```python
from build123d import *

# Parameters (mm, degrees)
BOSS_EXTRUDE1_DEPTH = 3.175
SKETCH2_R           = 1.5875
CUT_EXTRUDE_R_DEPTH = 216.549531721


with BuildPart() as part:
    # Sketch1 → Boss-Extrude1 (new body)
    with BuildSketch(Plane.XY):
        Polygon((0, 0), (0, 152.4), (152.4, 152.4), align=None)
    extrude(amount=BOSS_EXTRUDE1_DEPTH)

    # Sketch2 → Cut-Extrude r (cut, through all)
    with BuildSketch(Plane.XY.offset(3.175)):
        with Locations((12.7, 139.7)):
            Circle(SKETCH2_R)
        with Locations((34.29, 139.7)):
            Circle(SKETCH2_R)
        with Locations((55.88, 139.7)):
            Circle(SKETCH2_R)
        with Locations((77.47, 139.7)):
            Circle(SKETCH2_R)
        with Locations((12.7, 118.11)):
            Circle(SKETCH2_R)
        with Locations((12.7, 96.52)):
            Circle(SKETCH2_R)
        with Locations((12.7, 74.93)):
            Circle(SKETCH2_R)
        with Locations((38.1, 114.3)):
            Circle(SKETCH2_R)
        with Locations((57.15, 114.3)):
            Circle(SKETCH2_R)
        with Locations((38.1, 95.25)):
            Circle(SKETCH2_R)
        with Locations((99.06, 139.7)):
            Circle(SKETCH2_R)
        with Locations((120.65, 139.7)):
            Circle(SKETCH2_R)
        with Locations((12.7, 53.34)):
            Circle(SKETCH2_R)
        with Locations((12.7, 31.75)):
            Circle(SKETCH2_R)
        with Locations((76.2, 114.3)):
            Circle(SKETCH2_R)
        with Locations((95.25, 114.3)):
            Circle(SKETCH2_R)
        with Locations((38.1, 76.2)):
            Circle(SKETCH2_R)
        with Locations((38.1, 57.15)):
            Circle(SKETCH2_R)
    extrude(amount=-CUT_EXTRUDE_R_DEPTH, mode=Mode.SUBTRACT)


solid = part.part
```
For this review, take the finished solid that the model builds, in its own axes (mm). Round coordinates to 2 decimals unless told otherwise and drop trailing zeros. Loops run counter-clockwise (first coordinate to the right, second up) from the corner with the lowest first, then second, coordinate; pieces in that order, holes last.
Q1. Add section A-A on z = 0.8. Give the number of separate pieces and of enclosed holes in the cut face, plus the area to 3 significant figures.
Result sheet:
separate pieces: 1
enclosed holes: 18
area: 11,500 mm2
Q2. Add section C-C on x = 128. Write out the cut boundary in (y, z) (3 decimals), plus the area to 3 significant figures.
Result sheet:
outline: (128, 0) - (152.4, 0) - (152.4, 3.175) - (128, 3.175) - close
area: 77.5 mm2
Q3. To check wall thickness, follow line 1 along Y through (x, z) = (55.88, 2.35); line 2 along X through (y, z) = (96.52, 1.7); line 3 along Y through (x, z) = (77.47, 2.2). State the ranges of each line that lie inside material, in increasing order.
Result sheet:
line 1: y = 55.88 to 113.35, 115.25 to 138.11, 141.29 to 152.4
line 2: x = 0 to 11.11, 14.29 to 37.15, 39.05 to 96.52
line 3: y = 77.47 to 113.35, 115.25 to 138.11, 141.29 to 152.4
Q4. Add section B-B on y = 44. Write out the cut boundary in (x, z) (3 decimals).
Result sheet:
outline: (0, 0) - (44, 0) - (44, 3.175) - (0, 3.175) - close
Q5. Insertion check: pin 1 Ø1 at (x, z) = (37, 2.5) entering from -Y. The pin has a flat end and moves straight along its axis. Give the tip position at first contact, or say it passes through.
Result sheet:
pin 1: stops at y = 36.5
